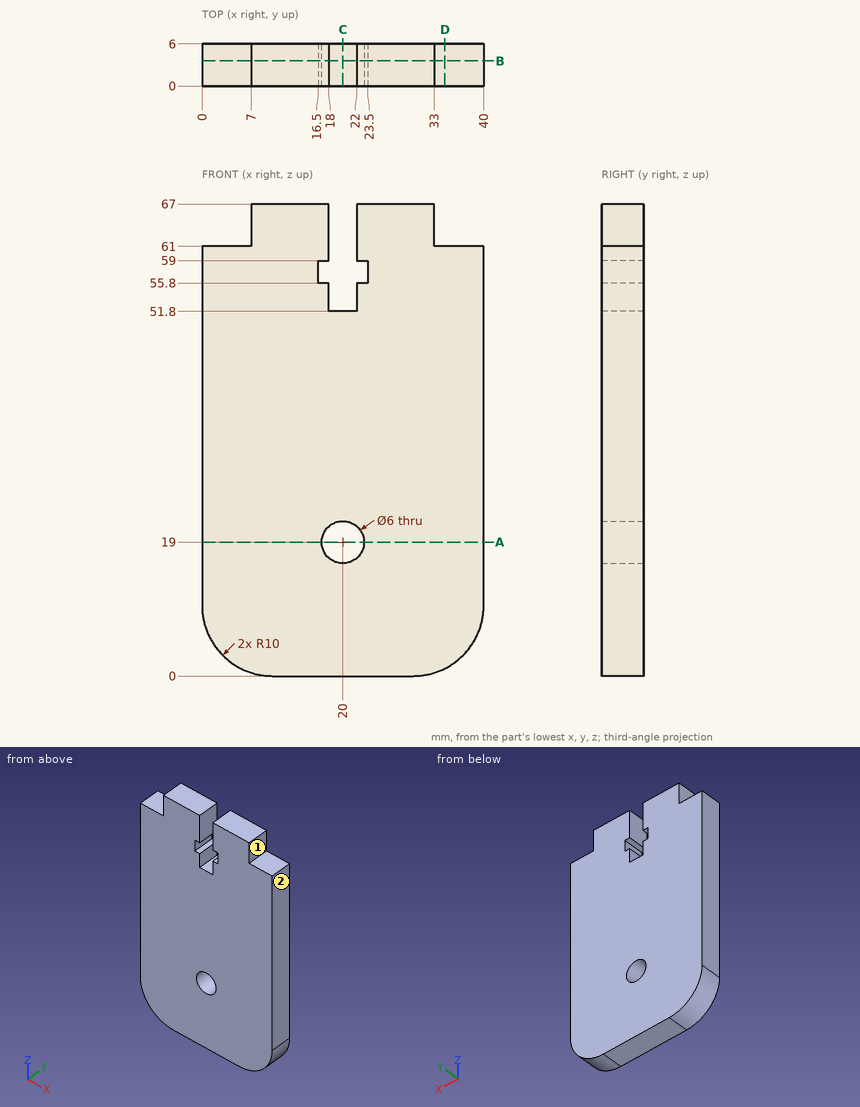
Input: dimensioned drawing with shaded views. Units: mm. Origin: part minimum x, y, z. A direction names the side the tool comes from. Give positions to 0.01 mm unless a question says otherwise; leave off trailing zeros. Loops run counter-clockwise (first coordinate to the right, second up) from the corner with the lowest first, then second, coordinate; pieces in that order, holes last. Notation, with made-up numbers: (75.5, 14) - (118.5, 14) arc R27 ccw to (118.5, 50) - close; hole circle Ø9 at (-15.75, 4). An arc over 180 degrees is marked (long way). Answer as CSV lines item,"result". Start each with the question number.
(1) Section query B-B (y = 3.6). Output: boundary loops of the cut face in (x, z), and give its area (3 significant figures).
(2) Section query D-D (x = 34.5). Output: boundary loops of the cut face in (y, z), and give its area (3 significant figures).
(3) Section query C-C (x = 20). Output: boundary loops of the cut face in (y, z), and give its area (3 significant figures).
(4) Section query A-A (z = 19). Output: boundary loops of the cut face in (x, y), and give its area (3 significant figures).
(5) Ray query, line 1 along Z through (x, y) = (20, 3.25); line 2 along Z through (x, y) = (17.5, 4.5); line 3 along X through (y, z) = (3.1, 19). Return the intervals inside material, ascending. Write a range as [from, to].
(6) Pin query (flat end, axial travel): P1, Ø6, axis at x = 19.5, z = 54.5, coming from the -Y side; P2, Ø1.8, axis at y = 3, z = 63, coming from the -X side; P3, Ø3, axis at x = 35, y = 3, coming from the +Z side. Return the tip coordinate at first contact, or that it passes through.
(7) Reachability of the marked faces 1 and 2 from +Z, -Z, +X, -X, +Y, -Y: full face, straight path, thin tool, end or side. Return the list, or none.
Worked answers:
1,outline,"(0, 10) arc R10 ccw to (10, 0) - (30, 0) arc R10 ccw to (40, 10) - (40, 61) - (33, 61) - (33, 67) - (22, 67) - (22, 59) - (23.5, 59) - (23.5, 55.8) - (22, 55.8) - (22, 51.8) - (18, 51.8) - (18, 55.8) - (16.5, 55.8) - (16.5, 59) - (18, 59) - (18, 67) - (7, 67) - (7, 61) - (0, 61) - close; hole circle Ø6 at (20, 19)"
1,area,"2,450 mm^2"
2,outline,"(0, 1.07) - (6, 1.07) - (6, 61) - (0, 61) - close"
2,area,"360 mm^2"
3,outline,"(0, 0) - (6, 0) - (6, 16) - (0, 16) - close; (0, 22) - (6, 22) - (6, 51.8) - (0, 51.8) - close"
3,area,"275 mm^2"
4,outline,"(0, 0) - (17, 0) - (17, 6) - (0, 6) - close; (23, 0) - (40, 0) - (40, 6) - (23, 6) - close"
4,area,"204 mm^2"
5,line 1,"z = [0, 16], [22, 51.8]"
5,line 2,"z = [0, 17.34], [20.66, 55.8], [59, 67]"
5,line 3,"x = [0, 17], [23, 40]"
6,P1,"stops at y = 0"
6,P2,"stops at x = 7"
6,P3,"stops at z = 61"
7,face 1,"+Z, +X, +Y, -Y"
7,face 2,"+Z, -Z, +X, +Y, -Y"
